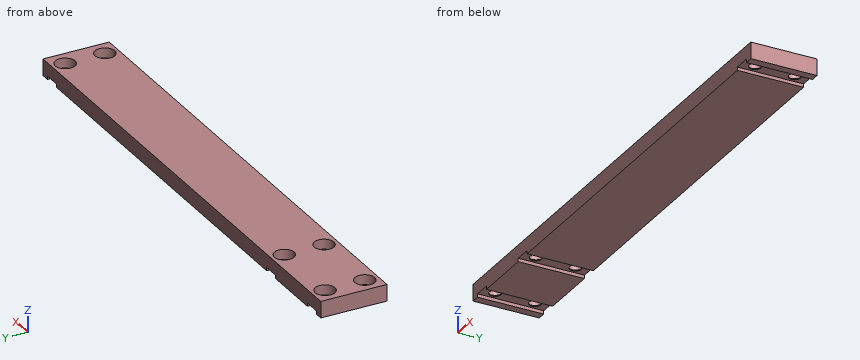
Autodesk Inventor part; units mm, degrees
ref_plane "YZ Plane" through (0, 0, 0) normal (1, 0, 0) x (0, 1, 0)
ref_plane "XZ Plane" through (0, 0, 0) normal (0, 1, 0) x (-1, 0, 0)
ref_plane "XY Plane" through (0, 0, 0) normal (0, 0, 1) x (1, 0, 0)
sketch "スケッチ1" plane through (0, 0, 0) normal (0, 0, 1) x (1, 0, 0)
  line L0 (0, 0) -> (155, 0)
  line L1 (155, 0) -> (155, 20)
  line L2 (155, 20) -> (0, 20)
  line L3 (0, 20) -> (0, 0)
  dimension "d0" = 155
  dimension "d1" = 20
extrude "押し出し1" add sketch "スケッチ1" along normal blind 5
sketch "スケッチ2" plane through (0, 0, 0) normal (0, 0, -1) x (-1, 0, 0)
  line L0 (-155, 0) -> (-155, 20)
  line L1 (0, 0) -> (-155, 0)
  line L2 (0, 20) -> (0, 0)
  line L3 (-155, 20) -> (0, 20)
  line L4 (-2.5, 20) -> (-7.5, 20)
  line L5 (-7.5, 20) -> (-7.5, 0)
  line L6 (-7.5, 0) -> (-2.5, 0)
  line L7 (-2.5, 0) -> (-2.5, 20)
  line L8 (-152.5, 0) -> (-147.5, 0)
  line L9 (-147.5, 0) -> (-147.5, 20)
  line L10 (-147.5, 20) -> (-152.5, 20)
  line L11 (-152.5, 20) -> (-152.5, 0)
  dimension "d4" = 5
  dimension "d5" = 2.5
  dimension "d6" = 5
  dimension "d7" = 2.5
extrude "押し出し2" cut sketch "スケッチ2" against normal blind 1 contours L11 L3 L9 L1 | L5 L3 L7 L1
sketch "スケッチ3" plane through (0, 0, 5) normal (0, -1, 0) x (1, 0, 0)
  line L0 (30.22, -4) -> (25.22, -4)
  line L1 (25.22, -4) -> (25.22, -356)
  line L2 (25.22, -356) -> (30.22, -356)
  line L3 (30.22, -356) -> (30.22, -4)
extrude "押し出し3" cut sketch "スケッチ3" against normal through all
sketch "スケッチ4" plane through (0, 0, 5) normal (0, 0, 1) x (1, 0, 0)
  circle A0 centre (5, 16) radius 1.2
  circle A1 centre (5, 4) radius 1.2
  circle A2 centre (27.72, 4) radius 1.2
  circle A3 centre (27.72, 16) radius 1.2
  circle A4 centre (150, 16) radius 1.2
  circle A5 centre (150, 4) radius 1.2
hole "穴1" at (5, 4, 5) at (5, 16, 5) at (27.72, 16, 5) at (27.72, 4, 5) at (150, 16, 5) at (150, 4, 5) direction (0, 0, -1) diameter 3.5 end through all
sketch "スケッチ5" plane through (0, 0, 5) normal (0, 0, 1) x (1, 0, 0)
  circle A0 centre (150, 16) radius 1.75
  circle A1 centre (27.72, 16) radius 1.75
  circle A2 centre (5, 4) radius 1.75
  circle A3 centre (5, 16) radius 1.75
  circle A4 centre (27.72, 4) radius 1.75
  circle A5 centre (150, 4) radius 1.75
hole "穴2" at (5, 4, 5) at (5, 16, 5) at (27.72, 4, 5) at (27.72, 16, 5) at (150, 16, 5) at (150, 4, 5) direction (0, 0, -1) diameter 6 depth 3 tip angle 118
properties part number "arm1_S" material "アルミニウム 6061"
Part model, mm, in its own coordinate system. Give positions to 0.01 mm unless a question says otherwise; leave off trailing zeros. Write each loop counter-clockwise with the first axis right and the second up, starting at its lowest first coordinate (ties: lowest second). Pieces come first, ordered by that corner, then holes. Notation, with made-up numbers: (-28.75, -23.75) -> (-6.75, -23.75) arc R23 cw to (-6.75, 3.25) -> close; hole circle Ø9 at (7.25, 2). An arc over 180 degrees is marked (long way). Put each result on its own line as item: value. Start each with the question number.
Item 1: Cut at B-B (z = 4). List the corners of the cut face in (x, y).
Item 2: Wall check: L1, parallel to Y at x = 150, z = 1.1; L2, parallel to X at y = 16, z = 0.3; L3, parallel to X at y = 4, z = 4.25. Give the ranges that are in metal, low to high. Write a range as [from, to].
Item 3: Cut at C-C (y = 4). State how many separate pieces and enclosed holes the cut face has, then the cut area to 3 significant figures.
Item 4: Cut at A-A (x = 150). List the corners of the cut face in (y, z), then the cut area to 3 significant figures.
Item 5: Pin check, flat tips, straight feed: pin 1 Ø1.1 at (y, z) = (10, 0.5) entering from -X; pin 2 Ø1.5 at (x, y) = (150, 6.5) entering from -Z; pin 3 Ø4.5 at (x, y) = (150, 4) entering from +Z. Stop position of each tip, or through.
Answer list:
1. outline: (0, 0) -> (155, 0) -> (155, 20) -> (0, 20) -> close; hole circle Ø6 at (5, 4); hole circle Ø6 at (5, 16); hole circle Ø6 at (27.72, 4); hole circle Ø6 at (27.72, 16); hole circle Ø6 at (150, 4); hole circle Ø6 at (150, 16)
2. L1: y = [0, 2.25], [5.75, 14.25], [17.75, 20]
2. L2: x = [0, 2.5], [7.5, 25.22], [30.22, 147.5], [152.5, 155]
2. L3: x = [0, 2], [8, 24.72], [30.72, 147], [153, 155]
3. separate pieces: 4
3. enclosed holes: 0
3. area: 693 mm2
4. outline: (0, 1) -> (2.25, 1) -> (2.25, 1.25) -> (1, 2) -> (1, 5) -> (0, 5) -> close; (5.75, 1) -> (14.25, 1) -> (14.25, 1.25) -> (13, 2) -> (13, 5) -> (7, 5) -> (7, 2) -> (5.75, 1.25) -> close; (17.75, 1) -> (20, 1) -> (20, 5) -> (19, 5) -> (19, 2) -> (17.75, 1.25) -> close
4. area: 35.1 mm2
5. pin 1: stops at x = 0
5. pin 2: stops at z = 1
5. pin 3: stops at z = 1.55
